Here's how the part is built. I have some questions about the finished solid (model axes, mm). A direction names the side the tool comes from. Coordinates: 2 decimals unless noted, no trailing zeros. Loops run counter-clockwise (first coordinate to the right, second up) from the corner with the lowest first, then second, coordinate; pieces in that order, holes last.
Autodesk Fusion 360 part; units mm, degrees
sketch "Sketch1" plane through (0, 0, 0) normal (0, 0, 1) x (1, 0, 0)
  line L0 (0, 0) -> (60, 0)
  line L1 (60, 0) -> (60, 10)
  line L2 (60, 10) -> (0, 10)
  line L3 (0, 10) -> (0, 0)
  dimension "d1" = 60
  dimension "d2" = 10
extrude "Extrude1" add sketch "Sketch1" along normal blind 2
hole "Hole1" at (55, 5, 2) direction (0, 0, -1) diameter 3.4 depth 8.6 tip angle 180 counterbore diameter 6.5 counterbore depth 3
sketch "Sketch2" plane through (0, 0, 0) normal (-1, 0, 0) x (0, -1, 0)
  line L0 (-10, 0) -> (0, 0)
  line L1 (0, 0) -> (0, 2)
  line L2 (0, 2) -> (-10, 2)
  line L3 (-10, 2) -> (-10, 0)
  line L4 (0, 2) -> (-10, 2)
  line L5 (-10, 2) -> (-10, 12)
  line L6 (-10, 12) -> (0, 12)
  line L7 (0, 12) -> (0, 2)
  dimension "d12" = 10
  dimension "d13" = 10
extrude "Extrude2" add sketch "Sketch2" against normal blind 10 contours L2 L4 L5 L6 L7
hole "Hole2" at (5, 0, 7) direction (0, 1, 0) diameter 6 depth 12 tip angle 180
sketch "Sketch3" plane through (0, 0, 2) normal (0, 0, 1) x (-1, 0, 0)
  line L0 (-10, -10) -> (-10, 0)
  line L1 (-10, 0) -> (-60, 0)
  line L2 (-60, 0) -> (-60, -10)
  line L3 (-60, -10) -> (-10, -10)
  circle A0 centre (-55, -5) radius 3.25
1. I need wall thicknesses on line 1 along Y through (x, z) = (55, 0.85); line 2 along X through (y, z) = (5.5, 7); line 3 along X through (y, z) = (5, 1.5). Which ranges of each line are inside material? Lowest first, please.
2. I want a section at C-C (z = 7). Please give me the cut outline in (x, y), then the cut area to 3 significant figures.
3. For pin 1 (5 mm diameter, centred on x = 25.5, y = 7.5, fed in from +Z); pin 2 (4 mm diameter, centred on y = 4.5, z = 7, fed in from +X), each with a flat end and sliding along its axis, tell me the tip position at first contact or that it passes through.
4. I want a section at B-B (x = 5). Please give me the cut outline in (y, z).
5. I want a section at D-D (y = 1.25). Please give me the cut outline in (x, z).
6. We'd pull the mould along Y, two halves only. Please class faces 1 (the flat face through (21, 10, 1.5)), 2 (the flat face through (19, 0, 1)), 3 (the cylindrical face through (51.778, 5.423, 0.986)), 4 (the flat face through (0, 5, 6)): +Y half, -Y half, draft (parallel to the pull), parting line (faces both ways), or undercut.
7. I want a section at A-A (y = 5). Please give me the cut outline in (x, z), then the cut area to 3 significant figures.
8. On a 3-axis mill with a long thin cutter (end or side, diameter ignored), from which of +Z, -Z, +X, -X, +Y, -Y can I reach the whole of each face in a straight line? I mean faces 5 (the flat face through (60, 5, 1)), 6 (the flat face through (10, 5, 7)). Say none if no direction works.
Response values:
1. line 1: y = 0 to 1.75, 8.25 to 10
1. line 2: x = 0 to 2, 8 to 10
1. line 3: x = 0 to 51.75, 58.25 to 60
2. outline: (0, 0) - (2, 0) - (2, 10) - (0, 10) - close; (8, 0) - (10, 0) - (10, 10) - (8, 10) - close
2. area: 40.0 mm2
3. pin 1: stops at z = 2
3. pin 2: stops at x = 10
4. outline: (0, 0) - (10, 0) - (10, 4) - (0, 4) - close; (0, 10) - (10, 10) - (10, 12) - (0, 12) - close
5. outline: (0, 0) - (60, 0) - (60, 2) - (10, 2) - (10, 12) - (0, 12) - close; hole circle Ø6 at (5, 7)
6. face 1: +Y half
6. face 2: -Y half
6. face 3: undercut
6. face 4: draft
7. outline: (0, 0) - (51.75, 0) - (51.75, 2) - (10, 2) - (10, 12) - (0, 12) - close; (58.25, 0) - (60, 0) - (60, 2) - (58.25, 2) - close; hole circle Ø6 at (5, 7)
7. area: 179 mm2
8. face 5: +Z, -Z, +X, +Y, -Y
8. face 6: +Z, +X, +Y, -Y
